```python
from build123d import *

# Parameters (mm, degrees)
F0_R     = 1.15
F1_DEPTH = 4
F0_W     = 4
F0_H     = 4
F2_DEPTH = 3.2
F4_START = -3
F3_W     = 10
F3_H     = 6
F4_DEPTH = 2


with BuildPart() as f1:
    # F0 (on Top) → F1 (new body, symmetric)
    with BuildSketch(Plane.XY):
        Circle(F0_R)
    extrude(amount=F1_DEPTH, both=True)

    # F0 (on Top) → F2 (join)
    with BuildSketch(Plane.XY):
        Rectangle(F0_W, F0_H)
        Circle(F0_R, mode=Mode.SUBTRACT)
        Circle(F0_R)
    extrude(amount=-F2_DEPTH)

    # F3 (on Top) → F4 (join)
    with BuildSketch(Plane.XY.offset(F4_START)):
        Rectangle(F3_W, F3_H)
    extrude(amount=-F4_DEPTH)


solid = f1.part
```
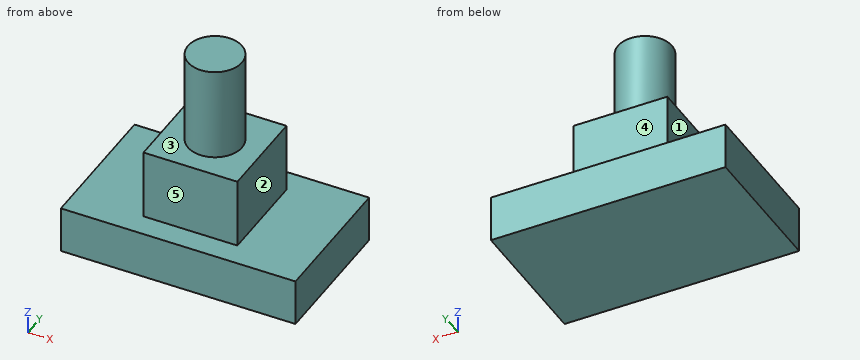
Build history of the part. All positions in model axes, mm. Face numbers are marked on the shaded views. A direction names the side the tool comes from. Give positions to 0.01 mm unless a question says otherwise; leave off trailing zeros. Loops run counter-clockwise (first coordinate to the right, second up) from the corner with the lowest first, then second, coordinate; pieces in that order, holes last. Notation, with made-up numbers: (87, 44.5) - (125, 44.5) arc R11 cw to (125, 50.5) - close; hole circle Ø3 at (65, 1.5). An arc over 180 degrees is marked (long way). Use a Markdown table: item, result.
(1) Band-saw the part on C-C (z = 0.5). Give the cut face in (x, y).
Taken from the geometry:
| item | result |
|---|---|
| outline | circle Ø2.3 at (0, 0) |
(2) Drop flat-ended pins along their axis: pin 1 Ø2 at (y, z) = (0.5, 2.5) entering from -X; pin 2 Ø3 at (x, z) = (0, -1) entering from -Y; pin 3 Ø3.5 at (y, z) = (0.5, -1) entering from -X. Give the stop position or say it passes through.
Taken from the geometry:
| item | result |
|---|---|
| pin 1 | x = -1.15 |
| pin 2 | y = -2 |
| pin 3 | x = -2 |
(3) Wall check: line 1 along Y through (x, z) = (1.75, -2.75); line 2 along Z through (x, y) = (4.5, 2.05); line 3 along Z through (x, y) = (1.25, -0.55). Give the ranges that are in metal, low to high.
Taken from the geometry:
| item | result |
|---|---|
| line 1 | -2 to 2 |
| line 2 | -5 to -3 |
| line 3 | -5 to 0 |
(4) Band-saw the part on B-B (y = 0). Give the cut face in (x, z).
Taken from the geometry:
| item | result |
|---|---|
| outline | (-5, -5) - (5, -5) - (5, -3) - (2, -3) - (2, 0) - (1.15, 0) - (1.15, 4) - (-1.15, 4) - (-1.15, 0) - (-2, 0) - (-2, -3) - (-5, -3) - close |
(5) Which spindle directions (+Z, -Z, +X, -X, +Y, -Y) get a long thin tool onto all of the face, cutting with end or side? Do the marked faces 1, 2, 3, 4 and 5. Say none if no direction does.
Taken from the geometry:
| item | result |
|---|---|
| face 1 | +Z, -X, +Y, -Y |
| face 2 | +Z, +X, +Y, -Y |
| face 3 | +Z |
| face 4 | +Z, +X, -X, +Y |
| face 5 | +Z, +X, -X, -Y |
(6) Band-saw the part on D-D (x = 0). Give the cut face in (y, z).
Taken from the geometry:
| item | result |
|---|---|
| outline | (-3, -5) - (3, -5) - (3, -3) - (2, -3) - (2, 0) - (1.15, 0) - (1.15, 4) - (-1.15, 4) - (-1.15, 0) - (-2, 0) - (-2, -3) - (-3, -3) - close |
(7) Band-saw the part on A-A (x = -1.75). Give the cut face in (y, z).
Taken from the geometry:
| item | result |
|---|---|
| outline | (-3, -5) - (3, -5) - (3, -3) - (2, -3) - (2, 0) - (-2, 0) - (-2, -3) - (-3, -3) - close |
